Verification items for the finished model (mm, model axes). Face numbers are marked on the shaded views. A direction names the side the tool comes from. Round coordinates to 2 decimals unless told otherwise and drop trailing zeros. Order: outer loops, then holes, each group sorted by start corner. A loop starts at its lowest first (then second) coordinate and runs counter-clockwise, first axis right, second up. Notation, with made-up numbers: (33, 60) -> (82, 60) arc R22 cw to (82, 72) -> close; hole circle Ø1 at (76, 27.5). An arc over 180 degrees is marked (long way). Return JSON: item names as keys, results as strings. Group by question number.
Item 1: Access from +Z, -Z, +X, -X, +Y, -Y to the whole of each face (thin tool, end or side, straight path). Record for the marked faces 1, 2 and 3.
Item 2: Sectioned sample at D-D on z = 31. Record the cut outline in (x, y), plus the area to 3 significant figures.
Item 3: Sectioned sample at B-B on x = 3. Record the cut outline in (y, z), plus the area to 3 significant figures.
Item 4: Draft check along X on the marked faces 4, 5, 6 and 7. Enter one of: pulls with the +X half, pulls with the -X half, needs draft (parallel to the pull), parting line crosses it, or undercut.
Item 5: Depth check by flat-ended pin: pin 1 Ø0.9 at (x, y) = (-27, 2.5) entering from -Z; pin 2 Ø4 at (x, y) = (-16.5, 66) entering from +Z; pin 3 Ø5 at (y, z) = (95.5, -4) entering from -X. Enter the tip coordinate at first touch or a pass-through.
Item 6: Sectioned sample at A-A on y = 127. Record the cut outline in (x, z).
Item 7: Sectioned sample at C-C on z = -15. Record the cut outline in (x, y).
Item 8: Scan lines: probe 1 along Y at (x, z) = (-21.5, 27.5); probe 2 along X at (y, z) = (103, -1); probe 3 along X at (y, z) = (119, -2). Record each from-to range of solid material in increasing order. Write a range as from..to.
```python
from build123d import *

# Parameters (mm, degrees)
BOSS_EXTRUDE1_DEPTH = 8
BOSS_EXTRUDE3_DEPTH = 127
SKETCH8_R           = 2.667
CUT_EXTRUDE1_DEPTH  = 127


with BuildPart() as part:
    # Sketch2 → Boss-Extrude1 (new body)
    with BuildSketch(Plane(origin=(0, 0, 0), x_dir=(1, 0, 0), z_dir=(0, 1, 0))):
        with BuildLine():
            ThreePointArc((-28.398063314, 25.4), (-26.940768363, -26.940768363), (25.4, -28.398063314))
            Line((25.4, -28.398063314), (25.4, -25.4))
            Line((25.4, -25.4), (28.398063314, -25.4))
            ThreePointArc((28.398063314, -25.4), (26.940768363, 26.940768363), (-25.4, 28.398063314))
            Line((-25.4, 28.398063314), (-25.4, 25.4))
            Line((-25.4, 25.4), (-28.398063314, 25.4))
        make_face()
        Polygon((10, 5.773502692), (10, -5.773502692), (0, -11.547005384), (-10, -5.773502692), (-10, 5.773502692), (0, 11.547005384), align=None, mode=Mode.SUBTRACT)
    extrude(amount=BOSS_EXTRUDE1_DEPTH)

    # Sketch7 → Boss-Extrude3 (add)
    with BuildSketch(Plane(origin=(0, 8, 0), x_dir=(1, 0, 0), z_dir=(0, 1, 0))):
        Polygon((-32.824735076, 2.610171349), (-14.307691077, -29.37771274), (-7.659250908, -25.529084967), (-26.176294907, 6.458799122), align=None)
    boss_extrude3 = extrude(amount=BOSS_EXTRUDE3_DEPTH)

    # Mirror1: Boss-Extrude3 across plane
    add(boss_extrude3.mirror(Plane(origin=(-21.745710428, -1.979026449, -37.664675308), x_dir=(0.4999999999999996, 0, 0.8660254037844389), z_dir=(0.8660254037844389, 0, -0.4999999999999996))))

    # Sketch8 → Cut-Extrude1 (cut)
    with BuildSketch(Plane(origin=(23.485284585, 0, -13.523431686), x_dir=(-0.49900881712180367, 0, -0.8665969076997092), z_dir=(0.8665969076997092, 0, -0.49900881712180367))):
        with Locations((-14.202194794, 93.725)):
            Circle(SKETCH8_R)
        with Locations((14.245786586, 42.925)):
            Circle(SKETCH8_R)
    extrude(amount=-CUT_EXTRUDE1_DEPTH, mode=Mode.SUBTRACT)


solid = part.part
```
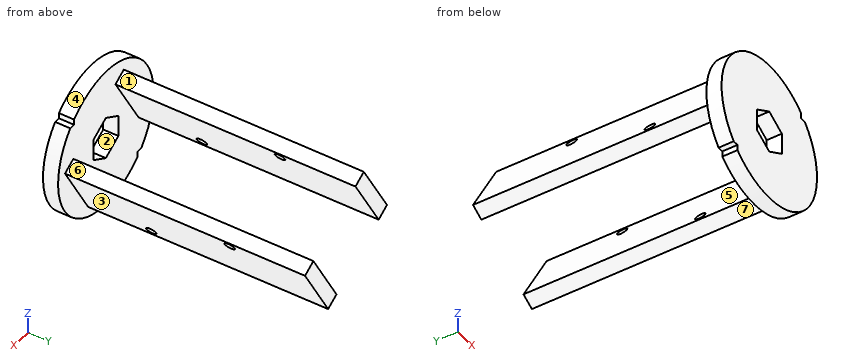
Recorded:
{
 "1": {"face 1": "+Z, +X, +Y", "face 2": "+Y, -Y", "face 3": "-Z, +X, +Y"},
 "2": {"outline": "(-22.15, 0) -> (22.15, 0) -> (22.15, 8) -> (-22.15, 8) -> close", "area": "354 mm²"},
 "3": {"outline": "(0, -37.98) -> (8, -37.98) -> (8, -9.81) -> (0, -9.81) -> close; (0, 9.81) -> (8, 9.81) -> (8, 37.98) -> (0, 37.98) -> close", "area": "451 mm²"},
 "4": {"face 4": "parting line crosses it", "face 5": "undercut", "face 6": "pulls with the +X half", "face 7": "pulls with the -X half"},
 "5": {"pin 1": "z = -25.4", "pin 2": "z = 29.05", "pin 3": "x = -32.82"},
 "6": {"outline": "(-32.82, -2.61) -> (-26.18, -6.46) -> (-7.66, 25.53) -> (-14.31, 29.38) -> close; (7.49, -25.9) -> (14.15, -29.73) -> (32.6, 2.3) -> (25.94, 6.13) -> close"},
 "7": {"outline": "(-35.02, 0) -> (35.02, 0) -> (35.02, 8) -> (22.64, 8) -> (22.64, 135) -> (13.77, 135) -> (13.77, 8) -> (-35.02, 8) -> close"},
 "8": {"probe 1": "0..8", "probe 2": "-31.89..-23.02, 21.83..30.7", "probe 3": "-32.47..-23.6, 21.26..30.12"}
}
